For this review, take the finished solid that the model builds, in its own axes (mm). Face numbers are marked on the shaded views. A direction names the side the tool comes from. Coordinates: 2 decimals unless noted, no trailing zeros. Loops run counter-clockwise (first coordinate to the right, second up) from the corner with the lowest first, then second, coordinate; pieces in that order, holes last.
1. Machinability: for the marked faces 1, 2 and 3, which of the approach directions +Z, -Z, +X, -X, +Y, -Y give a long, thin tool a straight path to every point of the face, cutting with its end or side? Answer none if there is none.
2. Take a section at B-B, the plane x = -0.5. State the section outline as (y, z) points, then the cut area to 3 significant figures.
3. Take a section at A-A, the plane x = 0. State the section outline as (y, z) points.
4. Take a section at C-C, the plane z = -8. State the section outline as (x, y) points (3 decimals), then the cut area to 4 significant figures.
5. To check wall thickness, follow probe 1 along Y at (x, z) = (0.3, -0.5). State the ranges of the line that lie inside material, in increasing order.
6. Clearance check with a flat-ended pin moving along its axis: P1, Ø0.5, axis at x = 0, y = -0.5, coming from the +Z side. State where the tip first meets the part, or that it passes through.
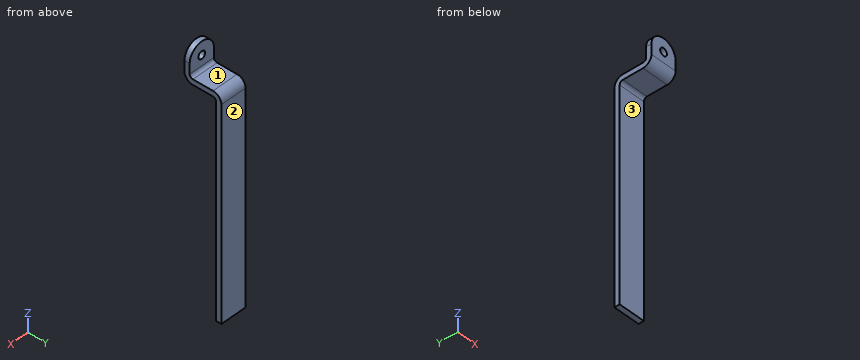
```python
from build123d import *

# Parameters (mm, degrees)
BASE_FLANGE1_DEPTH = 0.625
FILLET1_RADIUS     = 0.625
FILLET1_LENGTH     = 0.25
HOLE1_START        = -1.5
HOLE1_OUTLINE_R    = 0.175
HOLE1_DEPTH        = 0.25


# Read off the part's stored shape, not the designer's step: Hole1
# Sheet-metal steps are written as plain solids
with BuildPart() as part:
    # Sketch1 → Base-Flange1 (new, symmetric)
    with BuildSketch(Plane(origin=(0, 0, 0), x_dir=(0, 0, -1), z_dir=(1, 0, 0))):
        with BuildLine():
            Line((10, 0), (0.15, 0))
            ThreePointArc((0.15, 0), (0.043933983, -0.043933983), (0, -0.15))
            Line((0, -0.15), (0, -1.1))
            ThreePointArc((0, -1.1), (-0.117157288, -1.382842712), (-0.4, -1.5))
            Line((-0.4, -1.5), (-1.5, -1.5))
            Line((-1.5, -1.5), (-1.5, -1.25))
            Line((-1.5, -1.25), (-0.4, -1.25))
            ThreePointArc((-0.4, -1.25), (-0.293933983, -1.206066017), (-0.25, -1.1))
            Line((-0.25, -1.1), (-0.25, -0.15))
            ThreePointArc((-0.25, -0.15), (-0.132842712, 0.132842712), (0.15, 0.25))
            Line((0.15, 0.25), (10, 0.25))
            Line((10, 0.25), (10, 0))
        make_face()
    extrude(amount=BASE_FLANGE1_DEPTH, both=True)

    # Fillet1: full round fillet: the end face becomes a half cylinder, R = half its width
    fillet1_face = Plane((0, -1.375, 1.5), x_dir=(0, -1, 0), z_dir=(0, 0, 1))  # on the end face: x along it, z out of the body
    fillet1_slab = fillet1_face.offset(-FILLET1_RADIUS / 2) * Box(FILLET1_LENGTH, 2 * FILLET1_RADIUS, FILLET1_RADIUS, mode=Mode.PRIVATE)  # the body's end, R deep
    fillet1_round = Plane((0, -1.375, 0.875), x_dir=(0, 0, 1), z_dir=(0, -1, 0)) * Cylinder(FILLET1_RADIUS, FILLET1_LENGTH, mode=Mode.PRIVATE)  # its axis R under the face
    add(fillet1_slab - fillet1_round, mode=Mode.SUBTRACT)

    # Hole1 outline → Hole1 (cut)
    with BuildSketch(Plane(origin=(0, 0, 0), x_dir=(1, 0, 0), z_dir=(0, 1, 0)).offset(HOLE1_START)):
        with Locations((0.001471382, -0.886025874)):
            Circle(HOLE1_OUTLINE_R)
    extrude(amount=HOLE1_DEPTH, mode=Mode.SUBTRACT)


solid = part.part
```
Results list:
1. face 1: +Z, +X, -X, +Y
1. face 2: +Z, -Z, +X, -X, +Y
1. face 3: -Z, +X, -X, -Y
2. outline: (-1.5, 0.4) arc R0.4 ccw to (-1.1, 0) - (-0.15, 0) arc R0.15 cw to (0, -0.15) - (0, -10) - (0.25, -10) - (0.25, -0.15) arc R0.4 ccw to (-0.15, 0.25) - (-1.1, 0.25) arc R0.15 cw to (-1.25, 0.4) - (-1.25, 1.25) - (-1.5, 1.25) - close
2. area: 3.13 mm2
3. outline: (-1.5, 0.4) arc R0.4 ccw to (-1.1, 0) - (-0.15, 0) arc R0.15 cw to (0, -0.15) - (0, -10) - (0.25, -10) - (0.25, -0.15) arc R0.4 ccw to (-0.15, 0.25) - (-1.1, 0.25) arc R0.15 cw to (-1.25, 0.4) - (-1.25, 0.71) - (-1.5, 0.71) - close; (-1.5, 1.06) - (-1.25, 1.06) - (-1.25, 1.5) - (-1.5, 1.5) - close
4. outline: (-0.625, 0) - (0.625, 0) - (0.625, 0.25) - (-0.625, 0.25) - close
4. area: 0.3125 mm2
5. probe 1: y = 0 to 0.25
6. P1: stops at z = 0.25
